Can you work these out from the model? Positions are in its coordinate system, mm. A direction names the side the tool comes from. Coordinates: 2 decimals unless noted, no trailing zeros. Loops run counter-clockwise (first coordinate to the right, second up) from the corner with the lowest first, then second, coordinate; pieces in that order, holes last.
Autodesk Inventor part; units mm, degrees
ref_plane "YZ Plane" through (0, 0, 0) normal (1, 0, 0) x (0, 1, 0)
ref_plane "XZ Plane" through (0, 0, 0) normal (0, 1, 0) x (-1, 0, 0)
ref_plane "XY Plane" through (0, 0, 0) normal (0, 0, 1) x (1, 0, 0)
sketch "Sketch1" plane through (0, 0, 0) normal (0, 0, 1) x (1, 0, 0)
  line L0 (0, 0) -> (12.065, 0)
  line L1 (71.12, 0) -> (71.12, 9.398)
  line L2 (71.12, 9.398) -> (59.055, 9.398)
  line L3 (0, 9.398) -> (0, 0)
  circle A0 centre (7.62, 4.699) radius 1.6
  circle A1 centre (63.5, 4.699) radius 1.6
  line L4 (63.5, 4.699) -> (7.62, 4.699) construction
  line L5 (12.065, 9.398) -> (12.065, 0)
  line L6 (59.055, 0) -> (59.055, 9.398)
  line L7 (59.055, 9.398) -> (12.065, 9.398) construction
  line L8 (12.065, 9.398) -> (0, 9.398)
  line L9 (12.065, 0) -> (59.055, 0) construction
  line L10 (59.055, 0) -> (71.12, 0)
  line L11 (1.905, 9.398) -> (7.62, 4.699) construction
  line L12 (1.905, 0) -> (7.62, 4.699) construction
  line L13 (63.5, 4.699) -> (69.215, 9.398) construction
  line L14 (69.215, 0) -> (63.5, 4.699) construction
  line L15 (1.905, 0) -> (1.905, 9.398) construction
  line L16 (69.215, 0) -> (69.215, 9.398) construction
  line L17 (1.905, 0) -> (0, 9.398) construction
  line L18 (69.215, 0) -> (71.12, 9.398) construction
  dimension "d0" = 3.2
  dimension "d1" = 55.88
  dimension "d2" = 71.12
  dimension "d3" = 9.398
  dimension "d5" = 67.31
  dimension "d6" = 10.16
extrude "Extrusion1" add sketch "Sketch1" along normal blind 5
sketch "Sketch2" plane through (0, 0, 0) normal (0, -1, 0) x (1, 0, 0)
  circle A0 centre (35.56, 2.5) radius 38.735
  line L0 (0, 0) -> (12.065, 0) construction
  line L1 (12.065, 0) -> (12.065, 5) construction
  line L2 (0, 5) -> (12.065, 5) construction
  line L3 (0, 0) -> (0, 5) construction
  line L4 (71.12, 0) -> (59.055, 0) construction
  line L5 (71.12, 0) -> (71.12, 5) construction
  line L6 (59.055, 5) -> (71.12, 5) construction
  line L7 (59.055, 0) -> (59.055, 5) construction
  line L8 (12.065, 5) -> (35.56, 2.5) construction
  line L9 (71.12, 5) -> (59.055, 5)
  line L10 (35.56, 2.5) -> (59.055, 5) construction
  line L11 (59.055, 0) -> (71.12, 0)
  line L12 (59.055, 0) -> (35.56, 2.5) construction
  dimension "d9" = 77.47
extrude "Extrusion2" add sketch "Sketch2" along normal blind 6
sketch "Sketch3" plane through (0, 9.398, 0) normal (0, 1, 0) x (1, 0, 0)
  line L0 (1.905, -3.5) -> (69.215, -3.5)
  line L1 (69.215, -3.5) -> (69.215, -1.5)
  line L2 (69.215, -1.5) -> (1.905, -1.5)
  line L3 (1.905, -1.5) -> (1.905, -3.5)
  line L4 (71.12, 0) -> (59.055, 0) construction
  line L5 (69.215, -1.5) -> (71.12, 0) construction
  line L6 (71.0194, -5.1196) -> (69.215, -3.5) construction
  line L7 (0, 0) -> (0, -5) construction
  line L8 (0, -5) -> (1.905, -3.5) construction
  line L9 (1.905, -1.5) -> (0, 0) construction
  dimension "d12" = 67.31
  dimension "d13" = 2
extrude "Extrusion3" cut sketch "Sketch3" against normal up to surface (9.398 mm away)
fillet "Fillet1" radius 3.175 1 edges at (-3.175, 0, 2.5)
fillet "Fillet2" radius 3.175 8 edges at (12.065, 9.398, 4.25) (12.065, 9.398, 0.75) (12.065, 0, 4.25) (12.065, 0, 0.75) (59.055, 0, 0.75) (59.055, 9.398, 0.75) (59.055, 9.398, 4.25) (59.055, 0, 4.25)
properties part number "Base"
Item 1: I need wall thicknesses on line 1 along Y through (x, z) = (63.5, 0.75); line 2 along Y through (x, z) = (63, 4); line 3 along Y through (x, z) = (37, 20.5). Which ranges of each line are inside material? Lowest first, please.
Results are:
line 1: y = -6 to 3.1, 6.3 to 9.4
line 2: y = -6 to 3.18, 6.22 to 9.4
line 3: y = -6 to 0
Item 2: Suppose I cut it at C-C, the plane x = 35.56. Please give me the cut outline in (y, z) (3 decimals), plus the area to 3 significant figures.
Results are:
outline: (-6, -36.235) - (-3.175, -36.235) arc R3.175 ccw to (0, -33.06) - (0, 38.06) arc R3.175 ccw to (-3.175, 41.235) - (-6, 41.235) - close
area: 460 mm2
Item 3: Suppose I cut it at A-A, the plane y = 1.5. Please give me the cut outline in (x, z) (3 decimals).
Results are:
outline: (0, 0) - (12.543, 0) - (12.543, 1.5) - (1.905, 1.5) - (1.905, 3.5) - (12.543, 3.5) - (12.543, 5) - (0, 5) - close; (58.577, 0) - (71.12, 0) - (71.12, 5) - (58.577, 5) - (58.577, 3.5) - (69.215, 3.5) - (69.215, 1.5) - (58.577, 1.5) - close
Item 4: Suppose I cut it at B-B, the plane z = 2.5. Please give me the cut outline in (x, y) (3 decimals), plus the area to 3 significant figures.
Results are:
outline: (-3.175, -6) - (74.295, -6) - (74.295, -3.175) arc R3.175 ccw to (71.12, 0) - (71.12, 9.398) - (69.215, 9.398) - (69.215, 0) - (1.905, 0) - (1.905, 9.398) - (0, 9.398) - (0, 0) arc R3.175 ccw to (-3.175, -3.175) - close
area: 496 mm2
Item 5: We'd pull the mould along X, two halves only. Please class faces 6 (the face through (5, 9.398, 1)), 7 (the face through (7.412, 3.113, 0.74)), 8 (the face through (71.12, 5, 2)): +X half, -X half, draft (parallel to the pull), parting line (faces both ways), or undercut.
Results are:
face 6: draft
face 7: undercut
face 8: +X half
Item 6: Suppose I cut it at D-D, the plane x = 63.5. Count the separate pieces of the cut face and the enclosed holes in it, plus the area to 3 significant figures.
Results are:
separate pieces: 3
enclosed holes: 0
area: 334 mm2
Item 7: On a 3-axis mill with a long thin cutter (end or side, diameter ignored), from which of +Z, -Z, +X, -X, +Y, -Y can I reach the whole of each face in a straight line? I mean faces 1 (the face through (60.01, 8.493, 4.26)), 2 (the face through (69.215, 5, 3)), 3 (the face through (67, 9.398, 1)), 4 (the face through (72.506, -4.568, -9.135)), 5 (the face through (65.1, 3.7, 5)). Say none if no direction works.
Results are:
face 1: +Z, -Z, +Y
face 2: +Y
face 3: +Z, -Z, +X, -X, +Y
face 4: +Y, -Y
face 5: +Z, +X, -X, +Y
Item 8: I'm going to push flat-ended pins straight in: P1, Ø4, axis at x = 60, z = 19.5, coming from the +Y side; P2, Ø1, axis at y = -4, z = 25.5, coming from the +X side; P3, Ø1.2, axis at y = 5, z = 4.5, coming from the +X side; P4, Ø1, axis at y = 7, z = -1.5, coming from the -X side. Where does each tip first touch, or does it pass through?
Results are:
P1: stops at y = 0
P2: stops at x = 67.09
P3: stops at x = 71.12
P4: passes through
